Here's how the part is built. I have some questions about the finished solid (model axes, mm). Coordinates: 2 decimals unless noted, no trailing zeros. Write each loop counter-clockwise with the first axis right and the second up, starting at its lowest first coordinate (ties: lowest second). Pieces come first, ordered by that corner, then holes. Notation, with made-up numbers: (15, 16) - (58, 16) arc R27 ccw to (58, 35) - close; hole circle Ø8 at (-21, 56.25). An arc over 180 degrees is marked (long way). Answer in a Markdown table with one row per item. Add a question column.
Item 1: If I drill on probe 1 along X at (y, z) = (44, 3); probe 2 along X at (y, z) = (8, 1.75); probe 3 along Z at (x, y) = (-40, -45), over which ranges is the centre line in solid material (lowest first)? Write a range as from..to.
Item 2: I'm going to push flat-ended pins straight in: pin 1 (2 mm diameter, centred on y = -28, z = 2, fed in from +X); pin 2 (1.5 mm diameter, centred on y = 34.5, z = 4.5, fed in from +X). Where does each tip first touch, or does it pass through?
Item 3: Imagine slicing it at B-B (y = 30). Please give me the cut outline in (x, z), plus the area to 3 significant figures.
Item 4: Imagine slicing it at C-C (x = -31). Please give me the cut outline in (y, z), plus the area to 3 significant figures.
Item 5: Imagine slicing it at A-A (z = 3). Please give me the cut outline in (x, y), plus the area to 3 significant figures.
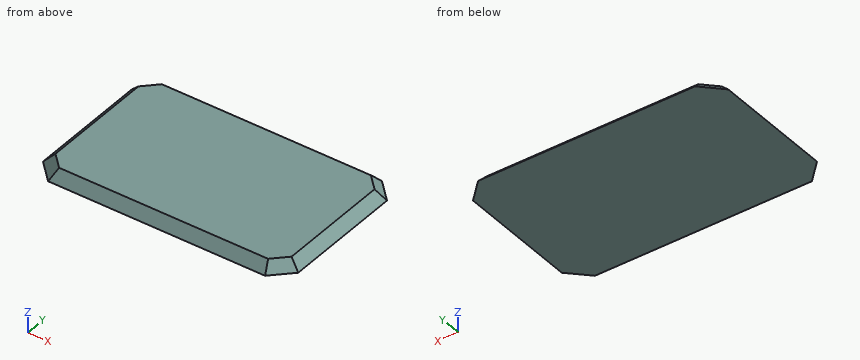
from build123d import *

# Parameters (mm, degrees)
SLOPED_45DEG_ROOF_FLAT_WEBCAM_TOP_DEPTH = 6
SLOPED_45DEG_ROOF_FLAT_WEBCAM_TOP_TAPER = 45


with BuildPart() as part:
    # Sketch1 → Sloped_45deg_Roof_Flat_Webcam_Top (new body)
    with BuildSketch(Plane.XY):
        Polygon((-78, -50), (58, -50), (70, -38), (70, 38), (58, 50), (-78, 50), (-90, 38), (-90, -38), align=None)
    extrude(amount=SLOPED_45DEG_ROOF_FLAT_WEBCAM_TOP_DEPTH, taper=SLOPED_45DEG_ROOF_FLAT_WEBCAM_TOP_TAPER)


solid = part.part
Here are the results:
| question | item | result |
|---|---|---|
| 1 | probe 1 | x = -79.76..59.76 |
| 1 | probe 2 | x = -88.25..68.25 |
| 1 | probe 3 | z = 0..5 |
| 2 | pin 1 | stops at x = 69 |
| 2 | pin 2 | stops at x = 66.25 |
| 3 | outline | (-90, 0) - (70, 0) - (64, 6) - (-84, 6) - close |
| 3 | area | 924 mm2 |
| 4 | outline | (-50, 0) - (50, 0) - (44, 6) - (-44, 6) - close |
| 4 | area | 564 mm2 |
| 5 | outline | (-87, -36.76) - (-76.76, -47) - (56.76, -47) - (67, -36.76) - (67, 36.76) - (56.76, 47) - (-76.76, 47) - (-87, 36.76) - close |
| 5 | area | 14,300 mm2 |
